from build123d import *

# Parameters (mm, degrees)
SKETCH2_R           = 2.1
BOSS_EXTRUDE1_DEPTH = 16
SKETCH3_R           = 2.1
BOSS_EXTRUDE2_DEPTH = 3
BOSS_EXTRUDE3_REACH = 21.35
SKETCH4_W           = 20
SKETCH4_H           = 3
FILLET1_R           = 10


with BuildPart() as part:
    # Sketch2 → Boss-Extrude1 (new body)
    with BuildSketch(Plane(origin=(0, 0, 0), x_dir=(0, 0, -1), z_dir=(1, 0, 0))):
        Circle(SKETCH2_R)
    extrude(amount=BOSS_EXTRUDE1_DEPTH)

    # Sketch3 → Boss-Extrude2 (add)
    with BuildSketch(Plane(origin=(16, 0, 0), x_dir=(0, 0, -1), z_dir=(1, 0, 0))):
        with Locations(Location((0, 0, 0), (0, 0, 270))):
            Circle(SKETCH3_R)
        with BuildLine():
            Line((3, 2.1), (0, 2.1))
            ThreePointArc((0, 2.1), (1.48492424, 1.48492424), (2.1, 0))
            ThreePointArc((2.1, 0), (1.48492424, -1.48492424), (0, -2.1))
            Line((0, -2.1), (3, -2.1))
            Line((3, -2.1), (3, 2.1))
        make_face()
    extrude(amount=BOSS_EXTRUDE2_DEPTH)

    # Boss-Extrude3: up to this face of the body (flat: up to its plane)
    boss_extrude3_end = Plane(part.part.faces().sort_by_distance((0, 0, 0))[0])
    # Sketch4 → Boss-Extrude3 (add, up to the picked face)
    with BuildSketch(Plane(origin=(19, 0, 0), x_dir=(0, 0, -1), z_dir=(1, 0, 0)), mode=Mode.PRIVATE) as boss_extrude3_sk1:
        with Locations((13, 0)):
            Rectangle(SKETCH4_W, SKETCH4_H)
    boss_extrude3_tool1 = split(extrude(boss_extrude3_sk1.sketch, amount=-BOSS_EXTRUDE3_REACH, mode=Mode.PRIVATE), bisect_by=boss_extrude3_end, keep=Keep.BOTH, mode=Mode.PRIVATE)
    add(boss_extrude3_tool1.solids().sort_by(Axis((19, 0, -13), (-1, 0, 0)))[0])

    # Fillet1
    # the kernel refuses this fillet: 10 mm, written as the material it adds along each edge
    with BuildSketch(Plane(origin=(19, -1.5, -3), x_dir=(0, -1, 0), z_dir=(-1, 0, 0))) as fillet1_piece_1:
        with BuildLine():
            CenterArc((10, -3.411744422), FILLET1_R, 160.051556411, 19.948443589)
            Line((0, -3.411744422), (0, 0))
            Line((0, 0), (0.6, 0))
        make_face()
    extrude(amount=3)
    with BuildSketch(Plane(origin=(19, 1.5, -3), x_dir=(0, 1, 0), z_dir=(-1, 0, 0))) as fillet1_piece_2:
        with BuildLine():
            CenterArc((10, 3.411744422), FILLET1_R, 180, 19.948443589)
            Line((0, 3.411744422), (0, 0))
            Line((0, 0), (0.6, 0))
        make_face()
    extrude(amount=3)


solid = part.part
Here's how the part is built. I have some questions about the finished solid (model axes, mm). A direction names the side the tool comes from. Round coordinates to 2 decimals unless told otherwise and drop trailing zeros. Order: outer loops, then holes, each group sorted by start corner. A loop starts at its lowest first (then second) coordinate and runs counter-clockwise, first axis right, second up. Notation, with made-up numbers: (39.25, 18) -> (90.25, 18) arc R7 ccw to (90.25, 23) -> close; hole circle Ø9 at (40.25, -35). An arc over 180 degrees is marked (long way). Return JSON: item names as keys, results as strings.
Q1. If we section it at C-C on z = -17.5: List the corners of the cut face in (x, y) for me, plus the area to 3 significant figures.
Filled sheet:
{"outline": "(0, -1.5) -> (19, -1.5) -> (19, 1.5) -> (0, 1.5) -> close", "area": "57.0 mm^2"}
Q2. If we section it at B-B on y = 0: List the corners of the cut face in (x, z) for me.
Filled sheet:
{"outline": "(0, -23) -> (19, -23) -> (19, 2.1) -> (0, 2.1) -> (0, -2.1) -> (16, -2.1) -> (16, -3) -> (0, -3) -> close"}
Q3. If we section it at A-A on x = 13: List the corners of the cut face in (y, z) for me.
Filled sheet:
{"outline": "circle Ø4.2 at (0, 0); (-1.5, -23) -> (1.5, -23) -> (1.5, -3) -> (-1.5, -3) -> close"}
Q4. Which directions (+Z, -Z, +X, -X, +Y, -Y) give clear straight access to the entire face, cutting with the end or side of a thin tool? Please do faces 1 (the cylindrical face through (17.521, -1.655, -4.656)), 2 (the cylindrical face through (9.37, 0.09, 2.1)).
Filled sheet:
{"face 1": "-Z, +X, -X, -Y", "face 2": "-X"}
Q5. If we mould it in two halves opening along Z, with no side actions, what happens to faces 3 (the flat face through (17, 2.1, -2)), 4 (the flat face through (10, 0, -23)), 5 (the flat face through (8, 0, -3))? For each: released by +Z, released by -Z, zero draft, split by the parting line, or undercut.
Filled sheet:
{"face 3": "zero draft", "face 4": "released by -Z", "face 5": "undercut"}
Q6. I need wall thicknesses on line 1 along Z through (x, y) = (8.5, 0.05); line 2 along Y through (x, z) = (14, -13); line 3 along Z through (x, y) = (3.25, 0.65). Which ranges of each line are inside material? Lowest first, please. Write a range as from..to.
Filled sheet:
{"line 1": "z = -23..-3, -2.1..2.1", "line 2": "y = -1.5..1.5", "line 3": "z = -23..-3, -2..2"}
Q7. For pin 1 Ø5.5 at (x, z) = (13.5, -12.5) entering from +Y, with a flat end and sliding along its axis, tell me the tip position at first contact or that it passes through.
Filled sheet:
{"pin 1": "stops at y = 1.5"}
